Here's how the part is built. I have some questions about the finished solid (model axes, mm). A direction names the side the tool comes from. Coordinates: 2 decimals unless noted, no trailing zeros. Order: outer loops, then holes, each group sorted by start corner. A loop starts at its lowest first (then second) coordinate and runs counter-clockwise, first axis right, second up. Notation, with made-up numbers: (-4.5, -4.75) - (17.5, -4.75) arc R37 cw to (17.5, 32.25) - close; hole circle Ø10 at (15, 50.25). An arc over 180 degrees is marked (long way). Use one line per item in the form item = value. Start each with the question number.
from build123d import *

# Parameters (mm, degrees)
SKETCH1_W               = 140
SKETCH1_H               = 70
BOSS_EXTRUDE1_DEPTH     = 45
CUT_EXTRUDE1_DEPTH      = 109.742815855
CUT_EXTRUDE1_DEPTH_BACK = 50
SKETCH2_W               = 140
SKETCH2_H               = 50
M10_CLEARANCE_HOLE1_D   = 10.5
CUT_EXTRUDE2_DEPTH      = 91.277350426
CUT_EXTRUDE2_DEPTH_BACK = 91.277350426
SKETCH9_W               = 12
SKETCH9_H               = 6
F_10_0MM_DOWEL_HOLE1_D  = 10
M8_TAPPED_HOLE1_D       = 6.8
M8_TAPPED_HOLE1_DEPTH   = 17.707073895
M8_TAPPED_HOLE1_TIP     = 2.042926105
M8_TAPPED_HOLE2_D       = 6.8
M8_TAPPED_HOLE2_DEPTH   = 17.707073895
M8_TAPPED_HOLE2_TIP     = 2.042926105


with BuildPart() as part:
    # Sketch1 → Boss-Extrude1 (new, symmetric)
    with BuildSketch(Plane.XY):
        Rectangle(SKETCH1_W, SKETCH1_H)
    extrude(amount=BOSS_EXTRUDE1_DEPTH, both=True)

    # Sketch2 → Cut-Extrude1 (cut, two sides: drawn at the far end of the back side and taken through both)
    with BuildSketch(Plane(origin=(0, 35, 0), x_dir=(1, 0, 0), z_dir=(0, 1, 0)).offset(-CUT_EXTRUDE1_DEPTH_BACK)):
        Rectangle(SKETCH2_W, SKETCH2_H)
    extrude(amount=CUT_EXTRUDE1_DEPTH + CUT_EXTRUDE1_DEPTH_BACK, mode=Mode.SUBTRACT)

    # M10 Clearance Hole1 (through all)
    with Locations(Plane(origin=(0, 35, 0), x_dir=(1, 0, 0), z_dir=(0, 1, 0))):
        with Locations((55, 35), (40, -35), (-25, -35), (-10, 35)):
            Hole(M10_CLEARANCE_HOLE1_D / 2)

    # Sketch9 → Cut-Extrude2 (cut, two sides: drawn at the far end of the back side and taken through both)
    with BuildSketch(Plane.XY.offset(-CUT_EXTRUDE2_DEPTH_BACK)):
        with Locations((-46, -32)):
            Rectangle(SKETCH9_W, SKETCH9_H)
    extrude(amount=CUT_EXTRUDE2_DEPTH + CUT_EXTRUDE2_DEPTH_BACK, mode=Mode.SUBTRACT)

    # Ø10.0mm Dowel Hole1 (through all)
    with Locations(Plane(origin=(0, 35, 0), x_dir=(1, 0, 0), z_dir=(0, 1, 0))):
        with Locations((55, -35), (-25, 35)):
            Hole(F_10_0MM_DOWEL_HOLE1_D / 2)

    # M8 Tapped Hole1
    with Locations(Plane(origin=(0, 35, 0), x_dir=(1, 0, 0), z_dir=(0, 1, 0))):
        with Locations((22.5, 35), (7.5, -35)):
            Hole(M8_TAPPED_HOLE1_D / 2, depth=M8_TAPPED_HOLE1_DEPTH)
            with Locations((0, 0, -(M8_TAPPED_HOLE1_DEPTH + M8_TAPPED_HOLE1_TIP / 2))):  # 118° drill point
                Cone(0, M8_TAPPED_HOLE1_D / 2, M8_TAPPED_HOLE1_TIP, mode=Mode.SUBTRACT)

    # M8 Tapped Hole2
    with Locations(Plane.ZY.offset(70)):
        with Locations((-35, 23), (-35, -23), (35, 23), (35, -23)):
            Hole(M8_TAPPED_HOLE2_D / 2, depth=M8_TAPPED_HOLE2_DEPTH)
            with Locations((0, 0, -(M8_TAPPED_HOLE2_DEPTH + M8_TAPPED_HOLE2_TIP / 2))):  # 118° drill point
                Cone(0, M8_TAPPED_HOLE2_D / 2, M8_TAPPED_HOLE2_TIP, mode=Mode.SUBTRACT)


solid = part.part
1) For pin 1 (5.5 mm diameter, centred on x = 22.5, z = -35, fed in from +Y), with a flat end and sliding along its axis, tell me the tip position at first contact or that it passes through.
2) Suppose I cut it at C-C, the plane x = -42.5. List the corners of the cut face in (y, z) for me.
3) Suppose I cut it at D-D, the plane z = 7.5. List the corners of the cut face in (x, y) for me, then the cut area to 3 significant figures.
4) Suppose I cut it at A-A, the plane y = 6. List the corners of the cut face in (x, z) for me.
5) Suppose I cut it at B-B, the plane x = -10. List the corners of the cut face in (y, z) for me.
6) If we mould it in two halves opening along Z, with no side actions, what happens to faces 5 (the flat face through (-40, -32, -1)), 6 (the flat face through (-1, 0, 45)), 7 (the cylindrical face through (-21.13, -0.49, 31.45))? For each: pulls with the +Z half, pulls with the -Z half, needs draft (parallel to the pull), parting line crosses it, or undercut.
7) Which directions (+Z, -Z, +X, -X, +Y, -Y) give clear straight access to the entire face, cutting with the end or side of a thin tool? Please do faces 1 (the flat face through (-52, -32, -1)), 2 (the flat face through (-1, -15, 0)), 3 (the cylindrical face through (4.36, 26.02, 36.3)), 4 (the cylindrical face through (-61.023, 24.021, 31.757)).
8) I need wall thicknesses on probe 1 along X at (y, z) = (30, -35); probe 2 along Z at (x, y) = (-59, -23); probe 3 along Y at (x, z) = (-60.5, -35). Which ranges of each line are inside material? Lowest first, please. Write a range as [from, to].
From the geometry:
q1.pin_1 = 16.9
q2.outline = (-29, -45) - (35, -45) - (35, -25) - (-15, -25) - (-15, 25) - (35, 25) - (35, 45) - (-29, 45) - close
q3.outline = (-70, -35) - (-52, -35) - (-52, -29) - (-40, -29) - (-40, -35) - (70, -35) - (70, -15) - (-70, -15) - close
q3.area = 2,730 mm2
q4.outline = (-70, -45) - (70, -45) - (70, -25) - (-70, -25) - close; (-70, 25) - (70, 25) - (70, 45) - (-70, 45) - close; hole circle Ø10.5 at (-25, 35); hole circle Ø10 at (-25, -35); hole circle Ø10.5 at (-10, -35); hole circle Ø10.5 at (40, 35); hole circle Ø10.5 at (55, -35); hole circle Ø10 at (55, 35)
q5.outline = (-35, -45) - (35, -45) - (35, -40.25) - (-35, -40.25) - close; (-35, -29.75) - (35, -29.75) - (35, -25) - (-15, -25) - (-15, 25) - (35, 25) - (35, 45) - (-35, 45) - close
q6.face_5 = needs draft
q6.face_6 = pulls with the +Z half
q6.face_7 = undercut
q7.face_1 = +Z, -Z, -Y
q7.face_2 = +X, -X, +Y
q7.face_3 = +Y
q7.face_4 = -X
q8.probe_1 = [-70, -30], [-20, -15.25], [-4.75, 19.1], [25.9, 49.75], [60.25, 70]
q8.probe_2 = [-45, -38.4], [-31.6, 31.6], [38.4, 45]
q8.probe_3 = [-35, -26.4], [-19.6, 19.6], [26.4, 35]
